from build123d import *

# Parameters (mm, degrees)
F0_W     = 381
F0_H     = 254
F1_DEPTH = 381
F2_W     = 279.4
F2_H     = 190.5
F3_DEPTH = 254.001
F4_W     = 279.4
F4_H     = 203.2
F5_DEPTH = 114.3


with BuildPart() as f1:
    # F0 (on Top) → F1 (new body)
    with BuildSketch(Plane.XY):
        Rectangle(F0_W, F0_H)
    extrude(amount=F1_DEPTH)

    # F2 (on face) → F3 (cut, through all)
    with BuildSketch(Plane.XZ.offset(127)):
        with Locations((0, 222.25)):
            Rectangle(F2_W, F2_H)
    extrude(amount=-F3_DEPTH, mode=Mode.SUBTRACT)

    # F4 (on face) → F5 (cut)
    with BuildSketch(Plane.XY.offset(127)):
        with Locations((0, 25.4)):
            Rectangle(F4_W, F4_H)
    extrude(amount=-F5_DEPTH, mode=Mode.SUBTRACT)


solid = f1.part
Geometry check sheet. Reference: the model listing, model coordinates, mm. A direction names the side the tool comes from. Round coordinates to 2 decimals unless told otherwise and drop trailing zeros. Write each loop counter-clockwise with the first axis right and the second up, starting at its lowest first coordinate (ties: lowest second). Pieces come first, ordered by that corner, then holes.
Item 1: Section check D-D (z = 97). Record the boundary of the cut face in (x, y), plus the area to 3 significant figures.
Determined:
outline: (-190.5, -127) - (190.5, -127) - (190.5, 127) - (139.7, 127) - (139.7, -76.2) - (-139.7, -76.2) - (-139.7, 127) - (-190.5, 127) - close
area: 40,000 mm2
Item 2: Section check B-B (z = 230). Record the boundary of the cut face in (x, y), plus the area to 3 significant figures.
Determined:
outline: (-190.5, -127) - (-139.7, -127) - (-139.7, 127) - (-190.5, 127) - close; (139.7, -127) - (190.5, -127) - (190.5, 127) - (139.7, 127) - close
area: 25,800 mm2
Item 3: Material ranges on line 1 along X through (y, z) = (-66.5, 242.5); line 2 along Z through (x, y) = (-53.5, 58); line 3 along Y through (x, z) = (116, 109.5), recorded low to high.
Determined:
line 1: x = -190.5 to -139.7, 139.7 to 190.5
line 2: z = 0 to 12.7, 317.5 to 381
line 3: y = -127 to -76.2
Item 4: Section check C-C (x = -116). Record the boundary of the cut face in (y, z), plus the area to 3 significant figures.
Determined:
outline: (-127, 0) - (127, 0) - (127, 12.7) - (-76.2, 12.7) - (-76.2, 127) - (-127, 127) - close; (-127, 317.5) - (127, 317.5) - (127, 381) - (-127, 381) - close
area: 25,200 mm2
Item 5: Mould release check, pull along X, two halves, no side actions. Record for faces 1 (the face through (190.5, -2, 188)), 2 (the face through (-1, 127, 331)), 3 (the face through (-2, -2, 317.5)): +X half, -X half, draft (parallel to the pull), parting line (faces both ways), or undercut.
Determined:
face 1: +X half
face 2: draft
face 3: undercut
Item 6: Section check A-A (y = -108.5). Record the boundary of the cut face in (x, z).
Determined:
outline: (-190.5, 0) - (190.5, 0) - (190.5, 381) - (-190.5, 381) - close; hole (-139.7, 127) - (139.7, 127) - (139.7, 317.5) - (-139.7, 317.5) - close
Item 7: Access from +Z, -Z, +X, -X, +Y, -Y to the whole of each face (thin tool, end or side, straight path). Record for faces 4 (the face through (-190.5, -2, 188)), 5 (the face through (-2, -102, 127)), 6 (the face through (139.7, -2, 163)).
Determined:
face 4: +Z, -Z, -X, +Y, -Y
face 5: +Y, -Y
face 6: +Y
Item 8: Go/stop test with flat-tipped pins: pin 1 Ø12 at (x, y) = (-125.5, -77) entering from -Z; pin 2 Ø2 at (x, z) = (118.5, 68) entering from +Y. Record where each tip stops, or that it passes through.
Determined:
pin 1: stops at z = 0
pin 2: stops at y = -76.2
